Could you check a few things on this drawing? It's one solid part, dimensions in mm from its lowest x, y, z. Give positions to 0.01 mm unless a question says otherwise; leave off trailing zeros. Write each loop counter-clockwise with the first axis right and the second up, starting at its lowest first coordinate (ties: lowest second). Pieces come first, ordered by that corner, then holes.
1. Suppose I cut it at A-A (y = 2.75). Please give me the cut outline in (x, z) (3 decimals).
2. Suppose I cut it at B-B (z = 0.85). Give the number of separate pieces and of enclosed holes in the cut face, and give its area (3 significant figures).
3. If I drill on probe 1 along X at (y, z) = (3.25, 0.2); probe 2 along X at (y, z) = (4.25, 1.35); probe 3 along Y at (x, z) = (40.5, 1.15), over which ranges is the centre line in solid material (lowest first)?
4. Suppose I cut it at D-D (x = 16). Please give me the cut outline in (y, z) (3 decimals).
5. Suppose I cut it at C-C (x = 3). Please give me the cut outline in (y, z) (3 decimals), and give its area (3 significant figures).
6. Thinking about a two-plate mould opening in Y: for the marked faces 1, 2 and 3, which applies, pulls with the +Y half, pulls with the -Y half, needs draft (parallel to the pull), parting line crosses it, or undercut?
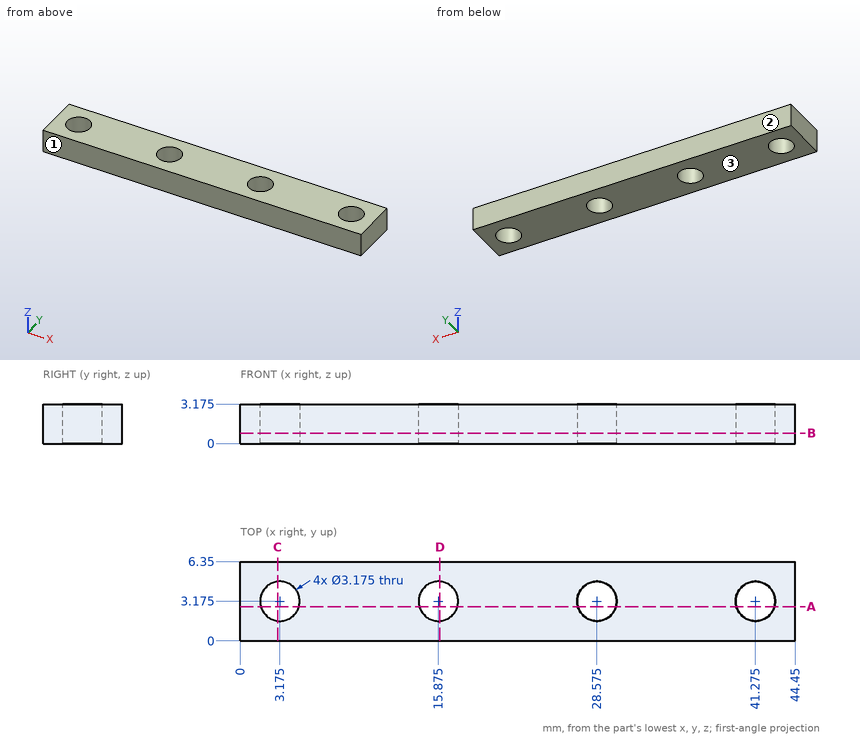
Checks:
1. outline: (0, 0) - (1.645, 0) - (1.645, 3.175) - (0, 3.175) - close; (4.705, 0) - (14.345, 0) - (14.345, 3.175) - (4.705, 3.175) - close; (17.405, 0) - (27.045, 0) - (27.045, 3.175) - (17.405, 3.175) - close; (30.105, 0) - (39.745, 0) - (39.745, 3.175) - (30.105, 3.175) - close; (42.805, 0) - (44.45, 0) - (44.45, 3.175) - (42.805, 3.175) - close
2. separate pieces: 1
2. enclosed holes: 4
2. area: 251 mm2
3. probe 1: x = 0 to 1.59, 4.76 to 14.29, 17.46 to 26.99, 30.16 to 39.69, 42.86 to 44.45
3. probe 2: x = 0 to 2.01, 4.34 to 14.71, 17.04 to 27.41, 29.74 to 40.11, 42.44 to 44.45
3. probe 3: y = 0 to 1.79, 4.56 to 6.35
4. outline: (0, 0) - (1.592, 0) - (1.592, 3.175) - (0, 3.175) - close; (4.758, 0) - (6.35, 0) - (6.35, 3.175) - (4.758, 3.175) - close
5. outline: (0, 0) - (1.597, 0) - (1.597, 3.175) - (0, 3.175) - close; (4.753, 0) - (6.35, 0) - (6.35, 3.175) - (4.753, 3.175) - close
5. area: 10.1 mm2
6. face 1: pulls with the -Y half
6. face 2: pulls with the +Y half
6. face 3: needs draft
